Here's how the part is built. I have some questions about the finished solid (model axes, mm). A direction names the side the tool comes from. Give positions to 0.01 mm unless a question says otherwise; leave off trailing zeros. Loops run counter-clockwise (first coordinate to the right, second up) from the corner with the lowest first, then second, coordinate; pieces in that order, holes last.
Q1. Suppose I cut it at A-A (z = 0). List the corners of the cut face in (x, y) for me, and give its area (3 significant figures).
Q2. Suppose I cut it at C-C (y = -10.5). List the corners of the cut face in (x, z) for me.
Q3. I'm going to push flat-ended pins straight in: P1, Ø4.5, axis at x = -11.5, y = 9, coming from the -Z side; P2, Ø1, axis at x = 12, y = 7, coming from the +Z side. Where does each tip first touch, or does it pass through?
Q4. Thinking about a two-plate mould opening in X: for faces 1 (the face through (26.833, -27.976, -23.049)), 2 (the face through (-3, 8, -28.937)), 3 (the face through (-32, -30.48, -29)), which applies, pulls with the +X half, pulls with the -X half, needs draft (parallel to the pull), parting line crosses it, or undercut?
Q5. Suppose I cut it at D-D (y = 7.62). Count the separate pieces of the cut face and the enclosed holes in it, and give its area (3 significant figures).
Q6. For faces 4 (the face through (44, 8, 28.937)), 5 (the face through (-32, -28, 21.317)), 6 (the face through (-30.505, -27.976, -24.009)), 7 (the face through (44, 8, -28.937)), 8 (the face through (26, -13, 28.937)), which set-ups out of +Z, -Z, +X, -X, +Y, -Y let a thin tool reach every point of the face, with its end or its side?
Q7. I need wall thicknesses on probe 1 along Z at (x, y) = (-46, 0.5); probe 2 along X at (y, z) = (2, 22); probe 3 along X at (y, z) = (-26, 29). Which ranges of each line are inside material? Lowest first, please.
Q8. Suppose I cut it at B-B (x = -19.5). List the corners of the cut face in (y, z) for me, and give its area (3 significant figures).
```python
from build123d import *

# Parameters (mm, degrees)
SKETCH1_W                = 117.5385
SKETCH1_H                = 57.8739
SKETCH1_W_2              = 109.6645
SKETCH1_H_2              = 47.7139
BOSS_EXTRUDE1_DEPTH      = 15.24
SKETCH2_R                = 1.97485
CUT_EXTRUDE1_DEPTH       = 129.032
SKETCH3_W                = 7.62
SKETCH3_H                = 7.62
BOSS_EXTRUDE2_DEPTH      = 30.48
BOSS_EXTRUDE2_DEPTH_BACK = 15.24
SKETCH4_W                = 7.62
SKETCH4_H                = 7.62
SKETCH4_R                = 1.545344409
SKETCH4_R_2              = 1.269040072
SKETCH4_R_3              = 1.671154259
SKETCH4_R_4              = 1.733603543
BOSS_EXTRUDE3_DEPTH      = 5.08


with BuildPart() as part:
    # Sketch1 → Boss-Extrude1 (new body)
    with BuildSketch(Plane(origin=(0, 0, 0), x_dir=(1, 0, 0), z_dir=(0, 1, 0))):
        Rectangle(SKETCH1_W, SKETCH1_H)
        Rectangle(SKETCH1_W_2, SKETCH1_H_2, mode=Mode.SUBTRACT)
    extrude(amount=BOSS_EXTRUDE1_DEPTH)

    # Sketch2 → Cut-Extrude1 (cut)
    with BuildSketch(Plane(origin=(58.76925, 0, 0), x_dir=(0, 0, -1), z_dir=(1, 0, 0))):
        with Locations((-13.4747, 7.62)):
            Circle(SKETCH2_R)
        with Locations((13.4747, 7.62)):
            Circle(SKETCH2_R)
    extrude(amount=-CUT_EXTRUDE1_DEPTH, mode=Mode.SUBTRACT)

    # Sketch3 → Boss-Extrude2 (add, two sides)
    with BuildSketch(Plane.XZ) as boss_extrude2_sk:
        with Locations((-32.09925, 32.74695)):
            Rectangle(SKETCH3_W, SKETCH3_H)
        with Locations((25.90074068, 32.74695)):
            Rectangle(SKETCH3_W, SKETCH3_H)
        with Locations((-32.09925, -32.74695)):
            Rectangle(SKETCH3_W, SKETCH3_H)
        with Locations((25.90074068, -32.74695)):
            Rectangle(SKETCH3_W, SKETCH3_H)
    extrude(amount=BOSS_EXTRUDE2_DEPTH)
    extrude(boss_extrude2_sk.sketch, amount=-BOSS_EXTRUDE2_DEPTH_BACK)

    # Sketch4 → Boss-Extrude3 (add)
    with BuildSketch(Plane.XZ.offset(30.48)):
        with Locations((-32.09925, 25.12695)):
            Rectangle(SKETCH4_W, SKETCH4_H)
        with Locations((-32.09925, 24.511)):
            Circle(SKETCH4_R, mode=Mode.SUBTRACT)
        with Locations((25.90074068, 25.12695)):
            Rectangle(SKETCH4_W, SKETCH4_H)
        with Locations((25.90074068, 24.511)):
            Circle(SKETCH4_R_2, mode=Mode.SUBTRACT)
        with Locations((-32.09925, -25.12695)):
            Rectangle(SKETCH4_W, SKETCH4_H)
        with Locations((-32.09925, -24.511)):
            Circle(SKETCH4_R_3, mode=Mode.SUBTRACT)
        with Locations((25.90074068, -25.12695)):
            Rectangle(SKETCH4_W, SKETCH4_H)
        with Locations((25.90074068, -24.511)):
            Circle(SKETCH4_R_4, mode=Mode.SUBTRACT)
    extrude(amount=-BOSS_EXTRUDE3_DEPTH)


solid = part.part
```
Solutions:
1. outline: (-58.77, 0) - (-54.83, 0) - (-54.83, 15.24) - (-58.77, 15.24) - close; (54.83, 0) - (58.77, 0) - (58.77, 15.24) - (54.83, 15.24) - close
1. area: 120 mm2
2. outline: (-35.91, -36.56) - (-28.29, -36.56) - (-28.29, -28.94) - (-35.91, -28.94) - close; (-35.91, 28.94) - (-28.29, 28.94) - (-28.29, 36.56) - (-35.91, 36.56) - close; (22.09, -36.56) - (29.71, -36.56) - (29.71, -28.94) - (22.09, -28.94) - close; (22.09, 28.94) - (29.71, 28.94) - (29.71, 36.56) - (22.09, 36.56) - close
3. P1: stops at z = -28.94
3. P2: stops at z = 28.94
4. face 1: undercut
4. face 2: undercut
4. face 3: needs draft
5. separate pieces: 4
5. enclosed holes: 0
5. area: 1,740 mm2
6. face 4: +Z, +X, +Y, -Y
6. face 5: +X, -X, +Y, -Y
6. face 6: -Y
6. face 7: -Z, +X, +Y, -Y
6. face 8: +X, -X
7. probe 1: z = -28.94 to -23.86, 23.86 to 28.94
7. probe 2: x = -58.77 to -54.83, 54.83 to 58.77
7. probe 3: x = -35.91 to -28.29, 22.09 to 29.71
8. outline: (0, -28.94) - (15.24, -28.94) - (15.24, -23.86) - (0, -23.86) - close; (0, 23.86) - (15.24, 23.86) - (15.24, 28.94) - (0, 28.94) - close
8. area: 155 mm2
